from build123d import *

# Parameters (mm, degrees)
SKETCH1_R           = 30
BOSS_EXTRUDE1_DEPTH = 15
SKETCH2_R           = 7.5
SKETCH2_R_2         = 1
BOSS_EXTRUDE2_DEPTH = 20
SKETCH4_R           = 3.175
CUT_EXTRUDE1_DEPTH  = 1.6
SKETCH5_W           = 2
SKETCH5_H           = 2.576429586
SKETCH5_W_2         = 1.5
SKETCH5_H_2         = 1
SKETCH5_4_W         = 1.5
SKETCH5_4_H         = 1
CUT_EXTRUDE2_START  = -5
SKETCH6_R           = 25
SKETCH6_R_2         = 10.076429586
CUT_EXTRUDE2_DEPTH  = 5
SKETCH7_R           = 25
CUT_EXTRUDE3_DEPTH  = 5
CUT_EXTRUDE4_START  = -5
CUT_EXTRUDE4_DEPTH  = 5
SKETCH9_W           = 1.5
SKETCH9_H           = 0.5


with BuildPart() as part:
    # Sketch1 → Boss-Extrude1 (new body)
    with BuildSketch(Plane.XY):
        Circle(SKETCH1_R)
    extrude(amount=BOSS_EXTRUDE1_DEPTH)

    # Sketch2 → Boss-Extrude2 (add)
    with BuildSketch(Plane.XY):
        Circle(SKETCH2_R)
        Circle(SKETCH2_R_2, mode=Mode.SUBTRACT)
    extrude(amount=-BOSS_EXTRUDE2_DEPTH)

    # Sketch4 → Cut-Extrude1 (cut)
    with BuildSketch(Plane(origin=(0, 0, -20), x_dir=(-1, 0, 0), z_dir=(0, 0, -1))):
        Circle(SKETCH4_R)
    extrude(amount=-CUT_EXTRUDE1_DEPTH, mode=Mode.SUBTRACT)

    # Sketch5 → Revolve2 (revolve)
    with BuildSketch(Plane(origin=(0, 0, 0), x_dir=(0, 0, -1), z_dir=(1, 0, 0)), mode=Mode.PRIVATE) as revolve2_sk:
        with Locations((1, 8.788214793)):
            Rectangle(SKETCH5_W, SKETCH5_H)
        with Locations((12.75, 7)):
            Rectangle(SKETCH5_W_2, SKETCH5_H_2)
    revolve(revolve2_sk.sketch.rotate(Axis((0, 0, -21.75), (0, 0, 1)), 270), axis=Axis((0, 0, -21.75), (0, 0, 1)))

    # Sketch5_4 → Cut-Revolve1 (revolve, cut)
    with BuildSketch(Plane(origin=(0, 0, 0), x_dir=(0, 0, -1), z_dir=(1, 0, 0)), mode=Mode.PRIVATE) as cut_revolve1_sk:
        with Locations((12.75, 7)):
            Rectangle(SKETCH5_4_W, SKETCH5_4_H)
    revolve(cut_revolve1_sk.sketch.rotate(Axis((0, 0, -21.75), (0, 0, 1)), 90), axis=Axis((0, 0, -21.75), (0, 0, 1)), mode=Mode.SUBTRACT)

    # Sketch6 → Cut-Extrude2 (cut)
    with BuildSketch(Plane(origin=(0, 0, 0), x_dir=(-1, 0, 0), z_dir=(0, 0, -1)).offset(CUT_EXTRUDE2_START)):
        Circle(SKETCH6_R)
        Circle(SKETCH6_R_2, mode=Mode.SUBTRACT)
    extrude(amount=CUT_EXTRUDE2_DEPTH, mode=Mode.SUBTRACT)

    # Sketch7 → Cut-Extrude3 (cut)
    with BuildSketch(Plane.XY.offset(15)):
        with Locations(Location((0, 0, 0), (0, 0, 180))):
            Circle(SKETCH7_R)
    extrude(amount=-CUT_EXTRUDE3_DEPTH, mode=Mode.SUBTRACT)

    # Sketch8 → Cut-Extrude4 (cut)
    with BuildSketch(Plane(origin=(0, 0, 5), x_dir=(-1, 0, 0), z_dir=(0, 0, -1)).offset(CUT_EXTRUDE4_START)):
        with BuildLine():
            Line((-10.076429586, 0), (-25, 0))
            ThreePointArc((-25, 0), (-24.388602599, 5.495094475), (-22.584314937, 10.721414032))
            Line((-22.584314937, 10.721414032), (-9.102770368, 4.321342942))
            ThreePointArc((-9.102770368, 4.321342942), (-9.830001471, 2.214837302), (-10.076429586, 0))
        make_face()
        with BuildLine():
            Line((-2.007140552, 24.919297478), (-0.808992418, 10.043901854))
            ThreePointArc((-0.808992418, 10.043901854), (-2.996895367, 9.620449644), (-5.038214793, 8.726444001))
            Line((-5.038214793, 8.726444001), (-12.5, 21.650635095))
            ThreePointArc((-12.5, 21.650635095), (-7.435409888, 23.868696651), (-2.007140552, 24.919297478))
        make_face()
        with BuildLine():
            Line((20.577174384, 14.197883446), (8.29377795, 5.722558913))
            ThreePointArc((8.29377795, 5.722558913), (6.833106104, 7.405612342), (5.038214793, 8.726444001))
            Line((5.038214793, 8.726444001), (12.5, 21.650635095))
            ThreePointArc((12.5, 21.650635095), (16.953192711, 18.373602176), (20.577174384, 14.197883446))
        make_face()
        with BuildLine():
            Line((22.584314937, -10.721414032), (9.102770368, -4.321342942))
            ThreePointArc((9.102770368, -4.321342942), (9.830001471, -2.214837302), (10.076429586, 0))
            Line((10.076429586, 0), (25, 0))
            ThreePointArc((25, 0), (24.388602599, -5.495094475), (22.584314937, -10.721414032))
        make_face()
        with BuildLine():
            Line((2.007140552, -24.919297478), (0.808992418, -10.043901854))
            ThreePointArc((0.808992418, -10.043901854), (2.996895367, -9.620449644), (5.038214793, -8.726444001))
            Line((5.038214793, -8.726444001), (12.5, -21.650635095))
            ThreePointArc((12.5, -21.650635095), (7.435409888, -23.868696651), (2.007140552, -24.919297478))
        make_face()
        with BuildLine():
            Line((-20.577174384, -14.197883446), (-8.29377795, -5.722558913))
            ThreePointArc((-8.29377795, -5.722558913), (-6.833106104, -7.405612342), (-5.038214793, -8.726444001))
            Line((-5.038214793, -8.726444001), (-12.5, -21.650635095))
            ThreePointArc((-12.5, -21.650635095), (-16.953192711, -18.373602176), (-20.577174384, -14.197883446))
        make_face()
    extrude(amount=CUT_EXTRUDE4_DEPTH, mode=Mode.SUBTRACT)

    # Sketch9 → Cut-Revolve2 (revolve, cut)
    with BuildSketch(Plane(origin=(0, 0, 0), x_dir=(0, 0, -1), z_dir=(1, 0, 0)), mode=Mode.PRIVATE) as cut_revolve2_sk:
        with Locations((-1.75, 29.75)):
            Rectangle(SKETCH9_W, SKETCH9_H)
        with Locations((-4.75, 29.75)):
            Rectangle(SKETCH9_W, SKETCH9_H)
        with Locations((-7.75, 29.75)):
            Rectangle(SKETCH9_W, SKETCH9_H)
        with Locations((-10.75, 29.75)):
            Rectangle(SKETCH9_W, SKETCH9_H)
        with Locations((-13.75, 29.75)):
            Rectangle(SKETCH9_W, SKETCH9_H)
    revolve(cut_revolve2_sk.sketch.rotate(Axis((0, 0, -21.75), (0, 0, 1)), 90), axis=Axis((0, 0, -21.75), (0, 0, 1)), mode=Mode.SUBTRACT)


solid = part.part
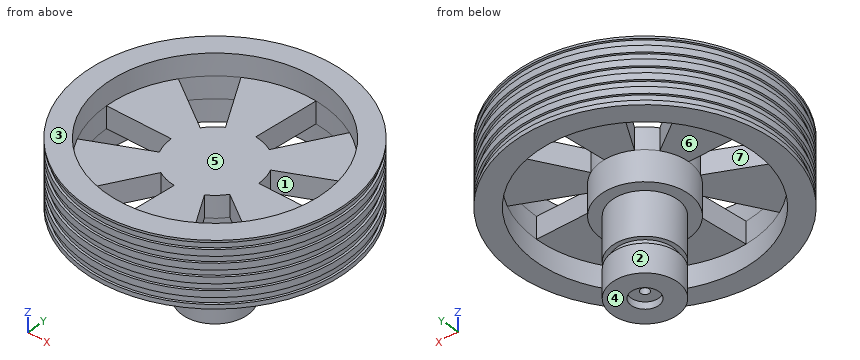
Work out the finished part from the listing and answer in its coordinate system (mm). Face numbers are marked on the shaded views. A direction names the side the tool comes from. Round coordinates to 2 decimals unless told otherwise and drop trailing zeros. Loops run counter-clockwise (first coordinate to the right, second up) from the corner with the lowest first, then second, coordinate; pieces in that order, holes last. Notation, with made-up numbers: (57, 56) -> (89, 56) arc R16 ccw to (89, 75) -> close; hole circle Ø4 at (-3.5, -34.75). An arc over 180 degrees is marked (long way). Use one line per item in the form item = value.
(1) Straight lines are drawn through the part: line 1 (Y direction, x = 0, z = 3.4); line 2 (Y direction, x = 0, z = 1.3); line 3 (Y direction, x = 0, z = -19) (3 decimals). For each, find the intervals that lie inside material, in ascending order.
Answer list:
line_1 = -30 to -25, -10.08 to 10.08, 25 to 30
line_2 = -29.5 to -25, -10.08 to 10.08, 25 to 29.5
line_3 = -7.5 to -3.175, 3.175 to 7.5
(2) Find section A-A on x = -18. Give the number of separate pieces and of enclosed holes in the cut face, then the cut area to 3 significant figures.
Answer list:
separate_pieces = 3
enclosed_holes = 0
area = 296 mm2
(3) For a pull along Y with two mould halves and no side action, classify the marked faces 1, 2 and 3 as released by +Y, released by -Y, zero draft, split by the parting line, or undercut.
Answer list:
face_1 = undercut
face_2 = split by the parting line
face_3 = zero draft
(4) A tool of negligible diameter and unlimited length cuts with its end or side. For the marked faces 4, 5, 6 and 7, from which of +Z, -Z, +X, -X, +Y, -Y can it reach the whole face along a straight path? Write none if from no direction.
Answer list:
face_4 = -Z, +X, -X, +Y, -Y
face_5 = +Z
face_6 = -Z
face_7 = +Z, -Z
(5) Find section C-C on z = -16. Give the vertices of the cut face in (x, y), then the cut area to 3 significant figures.
Answer list:
outline = circle Ø15 at (0, 0); hole circle Ø2 at (0, 0)
area = 174 mm2
(6) Flat-ended cylindrical pins translate along their axes: P1, Ø12, axis at y = 16.5, z = -2.5, coming from the +X side; P2, Ø7, axis at x = -0.5, y = -0.5, coming from the -Z side; P3, Ø4.5, axis at x = -5, y = 15.5, coming from the -Z side; P4, Ø12, axis at x = -3.5, y = 3.5, coming from the +Z side. Find the tip coordinate at first contact, or state that the pin passes through.
Answer list:
P1 = 27.89
P2 = -20
P3 = 5
P4 = 10
